Autodesk Inventor part; units mm, degrees
ref_plane "YZ Plane" through (0, 0, 0) normal (1, 0, 0) x (0, 1, 0)
ref_plane "XZ Plane" through (0, 0, 0) normal (0, 1, 0) x (-1, 0, 0)
ref_plane "XY Plane" through (0, 0, 0) normal (0, 0, 1) x (1, 0, 0)
sketch "Boceto1" plane through (0, 0, 0) normal (0, 0, 1) x (1, 0, 0)
  circle A0 centre (0, 0) radius 29
  dimension "Diametro" = 58
extrude "Extrusión1" add sketch "Boceto1" along normal blind 5
sketch "Boceto2" plane through (0, 0, 5) normal (0, 0, 1) x (1, 0, 0)
  circle A0 centre (1, -13.5) radius 1
  arc A1 (11.666, -9.2) -> (12.466, -10) centre (12.466, -9.2) ccw
  line L0 (5.15, -10.5) -> (-1.85, -10.5)
  circle A2 centre (9, -13.5) radius 1
  line L1 (5.15, 10.5) -> (5.15, -10.5)
  line L2 (25, 16) -> (25, -16)
  line L3 (25, -16) -> (-25, -16)
  line L4 (-25, 16) -> (25, 16)
  line L5 (-25, -16) -> (25, 16) construction
  line L6 (25, -16) -> (-25, 16) construction
  arc A3 (18.866, -4.8) -> (18.066, -4) centre (18.066, -4.8) ccw
  line L7 (18.066, -4) -> (12.466, -4)
  line L8 (12.466, -10) -> (18.066, -10)
  line L9 (15.266, -4) -> (12.466, -4)
  line L10 (11.666, -4.8) -> (11.666, -9.2)
  line L11 (18.866, -9.2) -> (18.866, -4.8)
  arc A4 (12.466, -4) -> (11.666, -4.8) centre (12.466, -4.8) ccw
  line L12 (-1.85, -10.5) -> (-1.85, 0)
  circle A5 centre (-7, -13.5) radius 1
  line L13 (-25, -16) -> (-25, 16)
  line L14 (-1.85, 0) -> (-1.85, 10.5)
  circle A6 centre (-13.5, 0) radius 6
  circle A7 centre (1, 13.5) radius 1
  line L15 (-1.85, 10.5) -> (5.15, 10.5)
  circle A8 centre (-7, 13.5) radius 1
  arc A9 (18.066, -10) -> (18.866, -9.2) centre (18.066, -9.2) ccw
  circle A10 centre (22.5, -8) radius 1
  circle A11 centre (17, -13.5) radius 1
  circle A12 centre (9, 13.5) radius 1
  arc A13 (12.466, 10) -> (11.666, 9.2) centre (12.466, 9.2) ccw
  line L16 (11.666, 4.8) -> (11.666, 9.2)
  arc A14 (11.666, 4.8) -> (12.466, 4) centre (12.466, 4.8) ccw
  circle A15 centre (17, 13.5) radius 1
  line L17 (15.266, 4) -> (12.466, 4)
  line L18 (12.466, 10) -> (18.066, 10)
  arc A16 (18.866, 9.2) -> (18.066, 10) centre (18.066, 9.2) ccw
  line L19 (18.066, 4) -> (15.266, 4)
  line L20 (18.866, 9.2) -> (18.866, 4.8)
  arc A17 (18.066, 4) -> (18.866, 4.8) centre (18.066, 4.8) ccw
  circle A18 centre (22.5, 8) radius 1
  point P0 (0, 0)
  dimension "d3" = 50
  dimension "d4" = 32
  dimension "d5" = 12
  dimension "d6" = 11.65
  dimension "d7" = 10.5
  dimension "d8" = 7
  dimension "d9" = 21
  dimension "d10" = 2.8
  dimension "d11" = 4.4
  dimension "d12" = 5.6
  dimension "d13" = 4.4
  dimension "d14" = 0.8
  dimension "d15" = 0.8
  dimension "d16" = 0.8
  dimension "d17" = 0.8
  dimension "d18" = 0.8
  dimension "d19" = 0.8
  dimension "d20" = 2
  dimension "d21" = 2
  dimension "d22" = 2
  dimension "d23" = 2
  dimension "d24" = 2
  dimension "d25" = 2
  dimension "d26" = 2
  dimension "d27" = 2
  dimension "d28" = 2
  dimension "d29" = 2
extrude "Extrusión2" cut sketch "Boceto2" against normal blind 3.2 contours L10 A4 L7 A3 L11 A9 L8 A1 | A6 | L18 A16 L20 A17 L19 L17 A14 L16 A13
extrude "Extrusión3" cut sketch "Boceto2" against normal blind 5 contours L0 L12 L14 L15 L1
sketch "Boceto3" plane through (0, 0, 5) normal (0, 0, 1) x (1, 0, 0)
  circle A0 centre (0, 0) radius 35
  circle A1 centre (0, 0) radius 29
  line L0 (0, 0) -> (22.6274, 22.6274)
  line L1 (0, 0) -> (32, 0) construction
  circle A2 centre (22.6274, 22.6274) radius 1.5
  circle A3 centre (-22.6274, 22.6274) radius 1.5
  circle A4 centre (-22.6274, -22.6274) radius 1.5
  circle A5 centre (22.6274, -22.6274) radius 1.5
  dimension "d34" = 70
  dimension "d35" = 58
  dimension "d40" = 32
  dimension "d41" = 45
  dimension "d42" = 3
  dimension "d45" = 360
extrude "Extrusión4" add sketch "Boceto3" against normal blind 3 contours A0 | A2 | A3 | A4 | A5
hole "Agujero1" at (22.6274, 22.6274, 5) at (-22.6274, 22.6274, 5) at (-22.6274, -22.6274, 5) at (22.6274, -22.6274, 5) direction (0, 0, -1) diameter 3.6881 depth 13
hole "Agujero2" at (-7, -13.5, 5) at (1, -13.5, 5) at (9, -13.5, 5) at (17, -13.5, 5) at (22.5, -8, 5) at (22.5, 8, 5) at (17, 13.5, 5) at (9, 13.5, 5) at (1, 13.5, 5) at (-7, 13.5, 5) direction (0, 0, -1) diameter 2.013 depth 7.6
equation "\"d35\" = Diametro"
properties part number "TE_01" material "PETG"
The listing builds one solid part. Answer for the finished solid, in the listing's coordinates (mm). A direction names the side the tool comes from. Coordinates: 2 decimals unless noted, no trailing zeros. Loops run counter-clockwise (first coordinate to the right, second up) from the corner with the lowest first, then second, coordinate; pieces in that order, holes last. Notation, with made-up numbers: M 49,-38 L 91,-38 A19 cw 91,-20 Z; hole C 58,-7 d7. An arc over 180 degrees is marked long. Answer in a Markdown table with one row per item.
1) Given pin 1 (2.5 mm diameter, centred on x = 16, z = 4, fed in from +Y); pin 2 (1.5 mm diameter, centred on x = -13, y = 4.5, fed in from +Z); pin 3 (4 mm diameter, centred on x = 22.63, y = -22.63, fed in from -Z); pin 4 (3.5 mm diameter, centred on x = -22.63, y = 22.63, fed in from -Z), each flat-ended and moving along its own axis, determine where each tip first touches the part or whether it passes through.
Answers below:
| item | result |
|---|---|
| pin 1 | y = 31.74 |
| pin 2 | z = 1.8 |
| pin 3 | z = 2 |
| pin 4 | through |
2) Determine the mould class of faces 4 (the flat face through (6, 0, 0)), 5 (the cylindrical face through (16.7, -14.46, 2.46)), 6 (the flat face through (2, -10.5, 3)) for opening direction Y: released by +Y, released by -Y, zero draft, split by the parting line, or undercut.
Answers below:
| item | result |
|---|---|
| face 4 | zero draft |
| face 5 | undercut |
| face 6 | undercut |
3) Find section A-A (y = 0). Determine the outline of the cut face in (x, z), then the cut area to 3 significant figures.
Answers below:
| item | result |
|---|---|
| outline | M -35,2 L -29,2 L -29,0 L -1.85,0 L -1.85,5 L -7.5,5 L -7.5,1.8 L -19.5,1.8 L -19.5,5 L -35,5 Z; M 5.15,0 L 29,0 L 29,2 L 35,2 L 35,5 L 5.15,5 Z |
| area | 253 mm^2 |
4) Find section B-B (x = 1). Determine the outline of the cut face in (y, z).
Answers below:
| item | result |
|---|---|
| outline | M -34.99,2 L -28.98,2 L -28.98,0 L -14.51,0 L -14.51,5 L -34.99,5 Z; M -12.49,0 L -10.5,0 L -10.5,5 L -12.49,5 Z; M 10.5,0 L 12.49,0 L 12.49,5 L 10.5,5 Z; M 14.51,0 L 28.98,0 L 28.98,2 L 34.99,2 L 34.99,5 L 14.51,5 Z |
5) Find section D-D (y = -13.5). Determine the outline of the cut face in (x, z).
Answers below:
| item | result |
|---|---|
| outline | M -32.29,2 L -25.67,2 L -25.67,0 L -8.01,0 L -8.01,5 L -32.29,5 Z; M -5.99,0 L -0.01,0 L -0.01,5 L -5.99,5 Z; M 2.01,0 L 7.99,0 L 7.99,5 L 2.01,5 Z; M 10.01,0 L 15.99,0 L 15.99,5 L 10.01,5 Z; M 18.01,0 L 25.67,0 L 25.67,2 L 32.29,2 L 32.29,5 L 18.01,5 Z |
6) Which of the six approach directions +Z, -Z, +X, -X, +Y, -Y give full straight-line access (tool end or side, diameter ignored) to faces 1 (the flat face through (5, 29, 2)), 2 (the flat face through (2, 10.5, 3)), 3 (the flat face through (-14, 0, 1.8))?
Answers below:
| item | result |
|---|---|
| face 1 | -Z |
| face 2 | +Z, -Z |
| face 3 | +Z |
7) Find the intervals of material crossed by probe 1 along X at (y, z) = (5.5, 2.15); probe 2 along X at (y, z) = (-7.5, 1.05); probe 3 along X at (y, z) = (-4.5, 2.6), in increasing order.
Answers below:
| item | result |
|---|---|
| probe 1 | -34.57 to -15.9, -11.1 to -1.85, 5.15 to 11.67, 18.87 to 34.57 |
| probe 2 | -28.01 to -1.85, 5.15 to 21.63, 23.37 to 28.01 |
| probe 3 | -34.71 to -17.47, -9.53 to -1.85, 5.15 to 11.72, 18.81 to 34.71 |
8) Find section C-C (y = 8). Determine the outline of the cut face in (x, z).
Answers below:
| item | result |
|---|---|
| outline | M -34.07,2 L -27.87,2 L -27.87,0 L -1.85,0 L -1.85,5 L -34.07,5 Z; M 5.15,0 L 21.49,0 L 21.49,5 L 18.87,5 L 18.87,1.8 L 11.67,1.8 L 11.67,5 L 5.15,5 Z; M 23.51,0 L 27.87,0 L 27.87,2 L 34.07,2 L 34.07,5 L 23.51,5 Z |
